CAD build for the part. Positions are in the model's coordinates, mm. Give positions to 0.01 mm unless a question says otherwise; leave off trailing zeros. Loops run counter-clockwise (first coordinate to the right, second up) from the corner with the lowest first, then second, coordinate; pieces in that order, holes last. Notation, with made-up numbers: M -19,-27 L 29,-27 A27 cw 29,-3 Z; hole C 35.5,-35 d11. An arc over 180 degrees is marked long. Answer as CSV lines item,"result".
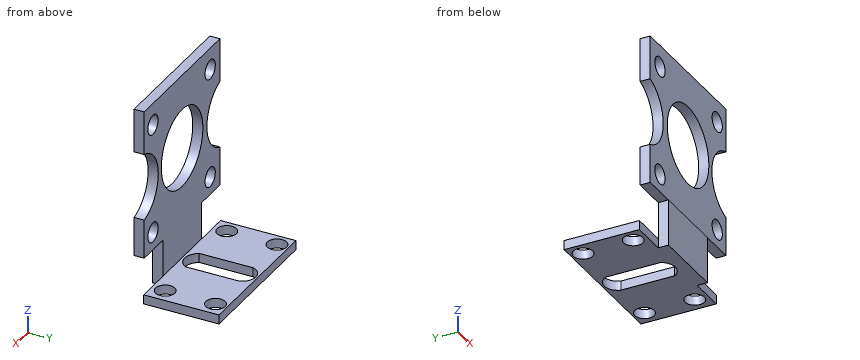
Autodesk Inventor part; units mm, degrees
ref_plane "YZ Plane" through (0, 0, 0) normal (1, 0, 0) x (0, 1, 0)
ref_plane "XZ Plane" through (0, 0, 0) normal (0, 1, 0) x (-1, 0, 0)
ref_plane "XY Plane" through (0, 0, 0) normal (0, 0, 1) x (1, 0, 0)
sketch "Sketch1" plane through (0, 0, 0) normal (0, 0, 1) x (1, 0, 0)
  line L0 (-10.9855, -5.6515) -> (10.9855, -5.6515)
  line L1 (10.9855, -5.6515) -> (10.9855, 5.6515)
  line L2 (10.9855, 5.6515) -> (-10.9855, 5.6515)
  line L3 (-10.9855, 5.6515) -> (-10.9855, -5.6515)
  line L4 (-10.9855, -5.6515) -> (10.9855, 5.6515) construction
  line L5 (10.9855, -5.6515) -> (-10.9855, 5.6515) construction
  point P0 (0, 0)
extrude "Extrusion1" add sketch "Sketch1" along normal blind 1.397
sketch "Sketch2" plane through (0, 0, 1.397) normal (0, 0, 1) x (1, 0, 0)
  circle A0 centre (-8.9011, 3.9017) radius 1.4605
  circle A1 centre (-8.9011, -3.6346) radius 1.4605
  circle A2 centre (8.6638, -3.6346) radius 1.4605
  circle A3 centre (8.6638, 3.9017) radius 1.4605
  line L0 (-2.0473, 3.9017) -> (-2.0473, -4.1687)
  line L1 (1.8989, 3.9017) -> (1.8989, -4.1687)
  arc A4 (1.8989, 3.9017) -> (-2.0473, 3.9017) centre (-0.0742, 3.3161) ccw
  arc A5 (-2.0473, -4.1687) -> (1.8989, -4.1687) centre (-0.0742, -3.0327) ccw
  point P0 (0, 0)
extrude "Extrusion2" cut sketch "Sketch2" against normal blind 25.4
sketch "Sketch3" plane through (0, 0, 0) normal (0, 1, 0) x (-1, 0, 0)
  point P0 (0, 0)
sketch "Sketch4" plane through (0, 0, 1.397) normal (0, 0, 1) x (1, 0, 0)
  line L0 (-2.0473, -4.1687) -> (-5.6033, -4.1687)
  line L1 (1.9681, -4.1687) -> (5.5241, -4.1687)
  line L2 (-10.9855, -5.6515) -> (10.9855, -5.6515)
  line L3 (-5.6033, -5.6515) -> (5.5241, -5.6515)
  line L4 (5.5241, -5.6515) -> (5.5241, -7.4092)
  line L5 (5.5241, -7.4092) -> (-5.6033, -7.4092)
  line L6 (-5.6033, -7.4092) -> (-5.6033, -5.6515)
  point P0 (0, 0)
  dimension "d11" = 3.556
  dimension "d12" = 3.556
extrude "Extrusion3" add sketch "Sketch4" along normal blind 5.5626 and the other way blind 1.397
sketch "Sketch6" plane through (-5.6033, -5.6515, 1.397) normal (0, 1, 0) x (1, 0, 0)
  line L0 (-5.1994, -5.5615) -> (-5.1994, -11.4289)
  line L1 (16.4285, -5.5615) -> (16.4285, -11.4289)
  arc A0 (-5.1994, -21.5321) -> (-5.1994, -11.4289) centre (-6.7732, -16.4805) ccw
  arc A1 (16.4285, -11.4289) -> (16.4285, -21.5321) centre (17.5971, -16.4805) ccw
  line L2 (16.4285, -21.5321) -> (16.4285, -28.1107)
  line L3 (-5.1994, -21.5321) -> (-5.1994, -28.1107)
  line L4 (-5.1994, -28.1107) -> (16.4285, -28.1107)
  circle A2 centre (5.6145, -16.911) radius 5.9336
  circle A3 centre (-2.4076, -8.2492) radius 1.4605
  circle A4 centre (13.9302, -8.2492) radius 1.4605
  circle A5 centre (-2.4076, -24.8214) radius 1.4605
  circle A6 centre (13.9302, -24.8214) radius 1.4605
  line L5 (-5.1994, -5.5615) -> (16.4285, -5.5615)
  point P0 (5.6033, 1.397)
  dimension "d20" = 2.921
  dimension "d21" = 2.921
  dimension "d22" = 2.921
  dimension "d23" = 2.921
extrude "Extrusion4" add sketch "Sketch6" against normal blind 1.524
sketch "Sketch8" plane through (-5.6033, -7.4092, 6.9596) normal (0, -1, 0) x (1, 0, 0)
  line L0 (11.1274, -5.5626) -> (11.1274, -6.9596)
  line L1 (0, 0) -> (0, -6.9596)
  line L2 (11.1274, -6.9596) -> (0, -6.9596)
  line L3 (0, -6.9596) -> (0, 0)
  line L4 (0, 0) -> (11.1274, 0)
  line L5 (11.1274, 0) -> (11.1274, -6.9596)
  point P0 (5.6033, -6.9596)
extrude "Extrusion5" cut sketch "Sketch8" against normal blind 0.2286
properties part number "motor mount"
Q1. Cut at D-D (x = 7.75). Write the cut outline in (y, z).
Solution:
outline,"M -7.18,6.96 L -5.65,6.96 L -5.65,8.3 L -7.18,8.3 Z; M -7.18,10.99 L -5.65,10.99 L -5.65,14.9 L -7.18,14.9 Z; M -7.18,20.86 L -5.65,20.86 L -5.65,24.88 L -7.18,24.88 Z; M -7.18,27.56 L -5.65,27.56 L -5.65,29.51 L -7.18,29.51 Z; M -5.65,0 L -4.77,0 L -4.77,1.4 L -5.65,1.4 Z; M -2.5,0 L 2.76,0 L 2.76,1.4 L -2.5,1.4 Z; M 5.04,0 L 5.65,0 L 5.65,1.4 L 5.04,1.4 Z"
Q2. Wall check: line 1 (Y direction, x = -6, z = 8); line 2 (Z direction, x = -5.5, y = -3.75); line 3 (Z direction, x = 3.5, y = -5.75). Give the ranges that are in metal, low to high. Write a range as [from, to].
Solution:
line 1,"y = [-7.18, -5.65]"
line 2,"z = [0, 1.4]"
line 3,"z = [0, 13.51], [23.11, 29.51]"
Q3. Pin check, flat tips, straight feed: P1, Ø3, axis at x = 6.5, z = 14.5, coming from the -Y side; P2, Ø3.5, axis at x = -4, y = 1.5, coming from the +Z side; P3, Ø0.5, axis at y = -6.5, z = 26, coming from the +X side; P4, Ø2.5, axis at x = 8.33, z = 9.65, coming from the -Y side. Stop position of each tip, or through.
Solution:
P1,"stops at y = -7.18"
P2,"stops at z = 1.4"
P3,"stops at x = 10.83"
P4,"passes through"
Q4. Cut at B-B (y = 0.5). Write the cut outline in (x, z).
Solution:
outline,"M -10.99,0 L -2.05,0 L -2.05,1.4 L -10.99,1.4 Z; M 1.9,0 L 10.99,0 L 10.99,1.4 L 1.9,1.4 Z"
Q5. Cut at C-C (z = 9). Write the cut outline in (x, y).
Solution:
outline,"M -10.8,-7.18 L -9.32,-7.18 L -9.32,-5.65 L -10.8,-5.65 Z; M -6.7,-7.18 L 7.02,-7.18 L 7.02,-5.65 L -6.7,-5.65 Z; M 9.64,-7.18 L 10.83,-7.18 L 10.83,-5.65 L 9.64,-5.65 Z"
